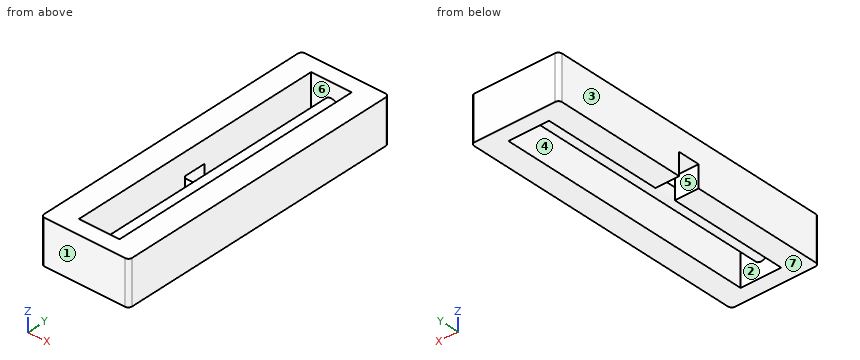
from build123d import *

# Parameters (mm, degrees)
F0_W     = 6
F0_H     = 20
F1_DEPTH = 3
F2_R     = 0.25
F3_W     = 2.773765591
F3_H     = 17.8463058546
F4_DEPTH = 5.9
F6_R     = 0.5
F7_DEPTH = 19.2
F8_W     = 1.5
F8_H     = 3
F9_DEPTH = 3.6


with BuildPart() as f1:
    # F0 (on Top) → F1 (new body)
    with BuildSketch(Plane.XY):
        Rectangle(F0_W, F0_H)
    extrude(amount=F1_DEPTH)

    # F2
    f2_edges = [f1.edges().sort_by_distance(p)[0] for p in [
        (3, 10, 1.5),
        (-3, 10, 1.5),
        (-3, -10, 1.5),
        (3, -10, 1.5),
    ]]
    fillet(f2_edges, radius=F2_R)

    # F3 (on Top) → F4 (cut)
    with BuildSketch(Plane.XY):
        with Locations((0.008794188, 0.008943025)):
            Rectangle(F3_W, F3_H)
    extrude(amount=F4_DEPTH, mode=Mode.SUBTRACT)

    # F6 (on offset) → F7 (join)
    with BuildSketch(Plane.XZ.offset(10)):
        with Locations((0, 1.5)):
            Circle(F6_R)
    extrude(amount=-F7_DEPTH)

    # F8 (on face) → F9 (cut)
    with BuildSketch(Plane.YZ.offset(-1.3780886075)):
        Rectangle(F8_W, F8_H)
    extrude(amount=-F9_DEPTH, mode=Mode.SUBTRACT)


solid = f1.part
The model under review builds one solid part; all positions refer to its coordinate system, in mm. Face numbers are marked on the shaded views. A direction names the side the tool comes from. Coordinates: 2 decimals unless noted, no trailing zeros. Loops run counter-clockwise (first coordinate to the right, second up) from the corner with the lowest first, then second, coordinate; pieces in that order, holes last. Notation, with made-up numbers: (82, 17.25) -> (128, 17.25) arc R15 ccw to (128, 30.25) -> close; hole circle Ø7 at (11.25, 37). An arc over 180 degrees is marked (long way). Use a Markdown table: item, result. Add a question column.
1. Add section A-A on y = 3.5. Write out the cut boundary in (x, z), plus the area to 3 significant figures.
2. Add section C-C on x = 0. Write out the cut boundary in (y, z).
3. Add section B-B on z = 2.25. Write out the cut boundary in (x, y), plus the area to 3 significant figures.
4. Machinability: for the marked faces 4, 5, 6 and 7, which of the approach directions +Z, -Z, +X, -X, +Y, -Y give a long, thin tool a straight path to every point of the face, cutting with its end or side? Answer none if there is none.
5. To check wall thickness, follow line 1 (Y direction, x = -0.35, z = 1.1); line 2 (X direction, y = -8.25, z = 0.8); line 3 (X direction, y = -7, z = 1.3). State the ranges of each line that lie inside material, in increasing order.
6. Clearance check with a flat-ended pin moving along its axis: pin 1 Ø0.8 at (x, y) = (-2, -0.5) entering from -Z. State where the tip first meets the part, or that it passes through.
7. Draft analysis for pull direction Y (two halves, no side actions). For the marked faces 1, 2 and 3, state which applies: pulls with the +Y half, pulls with the -Y half, needs draft (parallel to the pull), parting line crosses it, or undercut.
Returned:
| question | item | result |
|---|---|---|
| 1 | outline | (-3, 0) -> (-1.38, 0) -> (-1.38, 3) -> (-3, 3) -> close; circle Ø1 at (0, 1.5); (1.4, 0) -> (3, 0) -> (3, 3) -> (1.4, 3) -> close |
| 1 | area | 10.5 mm² |
| 2 | outline | (-10, 0) -> (-8.91, 0) -> (-8.91, 1) -> (8.93, 1) -> (8.93, 0) -> (10, 0) -> (10, 3) -> (8.93, 3) -> (8.93, 2) -> (-8.91, 2) -> (-8.91, 3) -> (-10, 3) -> close |
| 3 | outline | (-3, -9.75) arc R0.25 ccw to (-2.75, -10) -> (2.75, -10) arc R0.25 ccw to (3, -9.75) -> (3, 9.75) arc R0.25 ccw to (2.75, 10) -> (-2.75, 10) arc R0.25 ccw to (-3, 9.75) -> close; hole (-1.38, -8.91) -> (1.4, -8.91) -> (1.4, 8.93) -> (-1.38, 8.93) -> close |
| 3 | area | 70.4 mm² |
| 4 | face 4 | +Z, -Z |
| 4 | face 5 | -Z, -X |
| 4 | face 6 | none |
| 4 | face 7 | -Z, +X, -X, +Y, -Y |
| 5 | line 1 | y = -10 to -8.91, 8.93 to 10 |
| 5 | line 2 | x = -3 to -1.38, 1.4 to 3 |
| 5 | line 3 | x = -3 to -1.38, -0.46 to 0.46, 1.4 to 3 |
| 6 | pin 1 | stops at z = 0 |
| 7 | face 1 | pulls with the -Y half |
| 7 | face 2 | undercut |
| 7 | face 3 | needs draft |
